Here's how the part is built. I have some questions about the finished solid (model axes, mm). Face numbers are marked on the shaded views. Coordinates: 2 decimals unless noted, no trailing zeros. Order: outer loops, then holes, each group sorted by start corner. A loop starts at its lowest first (then second) coordinate and runs counter-clockwise, first axis right, second up. Notation, with made-up numbers: (55.25, 69) - (80.25, 69) arc R25 ccw to (80.25, 101) - close; hole circle Ø4 at (-8.75, 59.5). An arc over 180 degrees is marked (long way). Use CSV: the item, a comma, the result in double quotes. Start each with the question number.
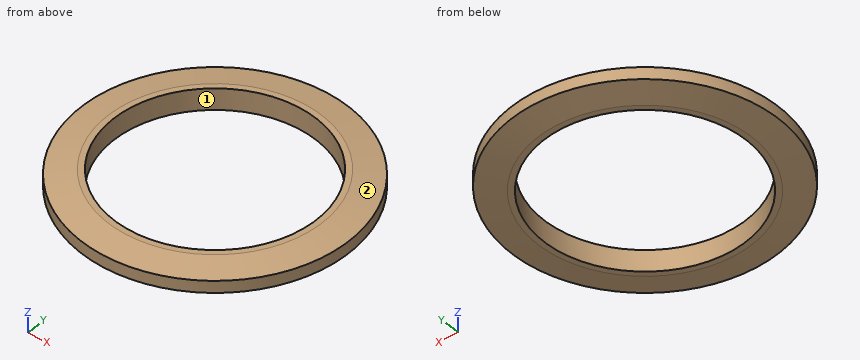
from build123d import *

# Parameters (mm, degrees)
SKETCH1_R           = 12.5
BOSS_EXTRUDE1_DEPTH = 2
SKETCH2_R           = 9.455
CUT_EXTRUDE1_DEPTH  = 2


with BuildPart() as part:
    # Sketch1 → Boss-Extrude1 (new body)
    with BuildSketch(Plane.XY):
        Circle(SKETCH1_R)
    extrude(amount=BOSS_EXTRUDE1_DEPTH)

    # Sketch2 → Cut-Extrude1 (cut)
    with BuildSketch(Plane.XY.offset(2)):
        Circle(SKETCH2_R)
    extrude(amount=-CUT_EXTRUDE1_DEPTH, mode=Mode.SUBTRACT)

    # Sketch3 → Cut-Revolve1 (revolve, cut)
    with BuildSketch(Plane(origin=(0, 0, 0), x_dir=(0, 0, -1), z_dir=(1, 0, 0)), mode=Mode.PRIVATE) as cut_revolve1_sk:
        Polygon((-2, 10), (-1.559182548, 12.5), (-2, 12.5), align=None)
        Polygon((-0.440817452, 12.5), (0, 12.5), (0, 10), align=None)
    revolve(cut_revolve1_sk.sketch.rotate(Axis((0, 0, -0.1), (0, 0, 1)), 90), axis=Axis((0, 0, -0.1), (0, 0, 1)), mode=Mode.SUBTRACT)


solid = part.part
Item 1: We'd pull the mould along X, two halves only. Please class the marked faces 1 and 2: released by +X, released by -X, zero draft, split by the parting line, or undercut.
Item 2: Please list where these lines run through material, in increasing order: line 1 along Y through (x, z) = (0, 0.5) (3 decimals); line 2 along X through (y, z) = (-8.5, 0.65); line 3 along Y through (x, z) = (-4, 1.2). Write a range as from..to.
Item 3: Suppose I cut it at A-A on y = 0. Write out the boundary of the cut face in (x, z) (3 decimals).
Item 4: For pin 1 Ø1 at (x, y) = (-6.5, -9) entering from +Z, with a flat end and sliding along its axis, tell me the tip position at first contact or that it passes through.
Here are the results:
1,face 1,"undercut"
1,face 2,"split by the parting line"
2,line 1,"-12.5..-9.455, 9.455..12.5"
2,line 2,"-9.17..-4.14, 4.14..9.17"
2,line 3,"-11.84..-8.57, 8.57..11.84"
3,outline,"(-12.5, 0.441) - (-10, 0) - (-9.455, 0) - (-9.455, 2) - (-10, 2) - (-12.5, 1.559) - close; (9.455, 0) - (10, 0) - (12.5, 0.441) - (12.5, 1.559) - (10, 2) - (9.455, 2) - close"
4,pin 1,"z = 1.89"
